from build123d import *

# Parameters (mm, degrees)
SKETCH4_W                    = 122.5
SKETCH4_H                    = 200
BOSS_EXTRUDE1_DEPTH          = 12
CUT_EXTRUDE1_DEPTH           = 12
FILLET1_R                    = 20
FILLET2_R                    = 20
FILLET3_R                    = 10
SKETCH10_R                   = 3.75
BOSS_EXTRUDE3_DEPTH          = 6
F_5_0_5_DIAMETER_HOLE1_D     = 5
F_5_0_5_DIAMETER_HOLE1_DEPTH = 8
F_5_0_5_DIAMETER_HOLE1_TIP   = 1.502151548
F_5_0_5_DIAMETER_HOLE2_D     = 5
F_5_0_5_DIAMETER_HOLE2_DEPTH = 8
F_5_0_5_DIAMETER_HOLE2_TIP   = 1.502151548


with BuildPart() as part:
    # Sketch4 → Boss-Extrude1 (new body)
    with BuildSketch(Plane.XY):
        with Locations((61.25, 100)):
            Rectangle(SKETCH4_W, SKETCH4_H)
    extrude(amount=BOSS_EXTRUDE1_DEPTH)

    # Sketch7 → Cut-Extrude1 (cut)
    with BuildSketch(Plane.XY.offset(12)):
        Polygon((43.985796602, 200), (122.5, 124.415794753), (122.5, 200), align=None)
    extrude(amount=-CUT_EXTRUDE1_DEPTH, mode=Mode.SUBTRACT)

    # Fillet1
    fillet1_edges = [part.edges().sort_by_distance(p)[0] for p in [
        (43.985796602, 200, 6),
    ]]
    fillet(fillet1_edges, radius=FILLET1_R)

    # Fillet2
    fillet2_edges = [part.edges().sort_by_distance(p)[0] for p in [
        (122.5, 124.415794753, 6),
    ]]
    fillet(fillet2_edges, radius=FILLET2_R)

    # Fillet3
    fillet3_edges = [part.edges().sort_by_distance(p)[0] for p in [
        (0, 200, 6),
    ]]
    fillet(fillet3_edges, radius=FILLET3_R)

    # Sketch10 → Boss-Extrude3 (add)
    with BuildSketch(Plane.XZ):
        with Locations(Location((26.25, 6, 0), (0, 0, 90))):
            Circle(SKETCH10_R)
        with Locations(Location((96.25, 6, 0), (0, 0, 90))):
            Circle(SKETCH10_R)
    extrude(amount=BOSS_EXTRUDE3_DEPTH)

    # Boss-Extrude4 cone 1 section (through the dimple's axis) → Boss-Extrude4 (revolve)
    with BuildSketch(Plane(origin=(26.25, -6, 6), x_dir=(0, 0, 1), z_dir=(1, 0, 0))):
        Polygon((0, 0), (3.75, 0), (0, 1.993910369), align=None)
    revolve(axis=Axis((26.25, -6, 6), (0, -1, 0)))

    # Boss-Extrude4 cone 2 section (through the dimple's axis) → Boss-Extrude4 cone 2 (revolve)
    with BuildSketch(Plane(origin=(96.25, -6, 6), x_dir=(0, 0, 1), z_dir=(1, 0, 0))):
        Polygon((0, 0), (3.75, 0), (0, 1.993910369), align=None)
    revolve(axis=Axis((96.25, -6, 6), (0, -1, 0)))

    # Ø5.0 (5) Diameter Hole1
    with Locations(Plane.ZY):
        with Locations((6, 180)):
            Hole(F_5_0_5_DIAMETER_HOLE1_D / 2, depth=F_5_0_5_DIAMETER_HOLE1_DEPTH)
            with Locations((0, 0, -(F_5_0_5_DIAMETER_HOLE1_DEPTH + F_5_0_5_DIAMETER_HOLE1_TIP / 2))):  # 118° drill point
                Cone(0, F_5_0_5_DIAMETER_HOLE1_D / 2, F_5_0_5_DIAMETER_HOLE1_TIP, mode=Mode.SUBTRACT)

    # Ø5.0 (5) Diameter Hole2
    with Locations(Plane.ZY):
        with Locations((6, 10)):
            Hole(F_5_0_5_DIAMETER_HOLE2_D / 2, depth=F_5_0_5_DIAMETER_HOLE2_DEPTH)
            with Locations((0, 0, -(F_5_0_5_DIAMETER_HOLE2_DEPTH + F_5_0_5_DIAMETER_HOLE2_TIP / 2))):  # 118° drill point
                Cone(0, F_5_0_5_DIAMETER_HOLE2_D / 2, F_5_0_5_DIAMETER_HOLE2_TIP, mode=Mode.SUBTRACT)


solid = part.part
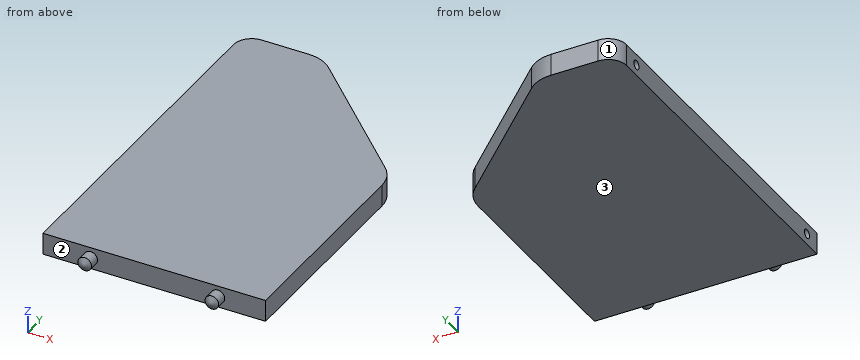
Build history of the part. All positions in model axes, mm. Face numbers are marked on the shaded views. Coordinates: 2 decimals unless noted, no trailing zeros. Order: outer loops, then holes, each group sorted by start corner. A loop starts at its lowest first (then second) coordinate and runs counter-clockwise, first axis right, second up. Notation, with made-up numbers: (40, 47.25) - (92, 47.25) arc R12 cw to (92, 57.25) - close; hole circle Ø3 at (37, 40.5). An arc over 180 degrees is marked (long way). Write each question's results on one line, items separated by ' | '. Start each with the question number.
Item 1: Wall check: probe 1 along Z at (x, y) = (5, 10); probe 2 along Y at (x, z) = (4.5, 6); probe 3 along Y at (x, z) = (2.5, 6). Give the ranges that are in metal, low to high. Write a range as [from, to].
Item 2: Mould opens along X. For the marked faces 1, 2 and 3 say: released by +X, released by -X, zero draft, split by the parting line, or undercut.
Item 3: Band-saw the part on A-A on x = 40. Write the cut outline in (y, z), and give its area (3 significant figures).
Item 4: Band-saw the part on B-B on y = 147. Write the cut outline in (x, z), and give its area (3 significant figures).
Item 5: Flat gauge pins, fed straight in: pin 1 (6 mm diameter, centred on x = 72, z = 8.5, fed in from -Y); pin 2 (5 mm diameter, centred on y = 119.5, z = 3.5, fed in from +X); pin 3 (2 mm diameter, centred on y = 162.5, z = 7.5, fed in from +X). Where does each tip first touch, or does it go through?
Numbers:
1) probe 1: [0, 3.5], [8.5, 12] | probe 2: [0, 7.5], [12.5, 177.5], [182.5, 198.35] | probe 3: [0, 7.5], [12.5, 177.5], [182.5, 196.61]
2) face 1: released by -X | face 2: undercut | face 3: zero draft
3) outline: (0, 0) - (199.58, 0) - (199.58, 12) - (0, 12) - close | area: 2,390 mm^2
4) outline: (0, 0) - (99.04, 0) - (99.04, 12) - (0, 12) - close | area: 1,190 mm^2
5) pin 1: y = 0 | pin 2: x = 122.47 | pin 3: x = 83.98
